Part model, mm, in its own coordinate system. A direction names the side the tool comes from. Give positions to 0.01 mm unless a question says otherwise; leave off trailing zeros. Order: outer loops, then holes, each group sorted by start corner. A loop starts at its lowest first (then second) coordinate and runs counter-clockwise, first axis right, second up. Notation, with made-up numbers: (38.5, 70) - (64.5, 70) arc R20 cw to (64.5, 105) - close; hole circle Ø5 at (18, 40.5). An arc over 180 degrees is marked (long way). Use one line per item in the form item = value. Start each with the question number.
1. Drill centre lines: line 1 (X direction, y = 5, z = -3.45); line 2 (Y direction, x = -25, z = -4.1); line 3 (X direction, y = 0, z = -2.4). Where is each one in solid material? Low to high.
2. Pull direction X, two halves, no side cores. Call faces 1 (the face through (-75, 0, 0)), 2 (the face through (-32.436, 5.976, 0.64)), 3 (the face through (1, 25, 0)): +X half, -X half, draft (parallel to the pull), parting line (faces both ways), or undercut.
3. Tool access for faces 4 (the face through (-69, -3, 2)), 5 (the face through (-1, -25, 0)): list every direction of +Z, -Z, +X, -X, +Y, -Y with a clear straight run to the whole face (end or side of a thin tool).
4. Band-saw the part on A-A, the plane x = -25. List the corners of the cut face in (y, z), plus the area to 3 significant figures.
5. Band-saw the part on B-B, the plane x = -45. List the corners of the cut face in (y, z), plus the area to 3 significant figures.
6. Pin check, flat tips, straight feed: P1, Ø8.5, axis at x = -45, y = 5, coming from the +Z side; P2, Ø24, axis at x = -25, y = 5, coming from the +Z side; P3, Ø7, axis at x = -65, y = 0, coming from the +Z side. Stop position of each tip, or through.
Autodesk Inventor part; units mm, degrees
ref_plane "YZ Plane" through (0, 0, 0) normal (1, 0, 0) x (0, 1, 0)
ref_plane "XZ Plane" through (0, 0, 0) normal (0, 1, 0) x (-1, 0, 0)
ref_plane "XY Plane" through (0, 0, 0) normal (0, 0, 1) x (1, 0, 0)
sketch "Sketch2" plane through (0, 0, 0) normal (0, 0, 1) x (1, 0, 0)
  line L0 (-75, -25) -> (75, -25)
  line L1 (75, -25) -> (75, 25)
  line L2 (75, 25) -> (-75, 25)
  line L3 (-75, 25) -> (-75, -25)
  line L4 (-75, -25) -> (75, 25) construction
  line L5 (75, -25) -> (-75, 25) construction
  point P0 (0, 0)
  dimension "d1" = 150
  dimension "d2" = 50
extrude "Extrusion1" add sketch "Sketch2" along normal mid plane 10
sketch "Sketch3" plane through (0, 0, 5) normal (0, 0, 1) x (1, 0, 0)
  line L0 (-75, 25) -> (-75, -25)
  line L1 (75, 25) -> (-75, 25)
  point P0 (0, 0)
  point P1 (-65, 0)
  dimension "d40" = 10
  dimension "d43" = 25
hole "Hole1" at (-65, 0, 5) direction (0, 0, -1) diameter 5.5 depth 14.2 tip angle 118 counterbore diameter 10 counterbore depth 5.4
sketch "Sketch4" plane through (0, 0, 5) normal (0, 0, 1) x (1, 0, 0)
  line L0 (-75, 25) -> (-75, -25)
  line L1 (75, 25) -> (-75, 25)
  point P0 (0, 0)
  point P1 (-45, 5)
  dimension "d41" = 30
  dimension "d42" = 20
hole "Hole2" at (-45, 5, 5) direction (0, 0, -1) diameter 6.6 depth 14.2 tip angle 118 counterbore diameter 11 counterbore depth 6.5
sketch "Sketch5" plane through (0, 0, 5) normal (0, 0, 1) x (1, 0, 0)
  line L0 (-75, 25) -> (-75, -25)
  line L1 (75, 25) -> (-75, 25)
  point P0 (0, 0)
  point P1 (-25, 5)
  dimension "d44" = 50
  dimension "d45" = 20
hole "Hole3" at (-25, 5, 5) direction (0, 0, -1) diameter 9 depth 14.2 tip angle 118 counterbore diameter 15 counterbore depth 8.6
properties part number "홀간 거리 확인 파트-6" material "SS400"
From the geometry:
q1.line_1 = -75 to -48.3, -41.7 to -32.5, -17.5 to 75
q1.line_2 = -25 to 0.5, 9.5 to 25
q1.line_3 = -75 to -67.75, -62.25 to -30.59, -19.41 to 75
q2.face_1 = -X half
q2.face_2 = undercut
q2.face_3 = draft
q3.face_4 = +Z
q3.face_5 = +Z, -Z, +X, -X, -Y
q4.outline = (-25, -5) - (0.5, -5) - (0.5, -3.6) - (-2.5, -3.6) - (-2.5, 5) - (-25, 5) - close; (9.5, -5) - (25, -5) - (25, 5) - (12.5, 5) - (12.5, -3.6) - (9.5, -3.6) - close
q4.area = 358 mm²
q5.outline = (-25, -5) - (1.7, -5) - (1.7, -1.5) - (-0.5, -1.5) - (-0.5, 5) - (-25, 5) - close; (8.3, -5) - (25, -5) - (25, 5) - (10.5, 5) - (10.5, -1.5) - (8.3, -1.5) - close
q5.area = 405 mm²
q6.P1 = -1.5
q6.P2 = 5
q6.P3 = -0.4
